Autodesk Inventor part; units mm, degrees
ref_plane "ba2_XY" through (19.05, 7.8105, 0) normal (0, 0, 1) x (1, 0, 0)
ref_plane "ba2_YZ" through (19.05, 7.8105, 0) normal (1, 0, 0) x (0, 1, 0)
ref_plane "ba2_ZX" through (19.05, 7.8105, 0) normal (0, 1, 0) x (0, 0, 1)
sketch "Sketch_1" plane through (0, 0, 0) normal (0, 0, 1) x (1, 0, 0)
  line L0 (29.3624, 0) -> (0, 0)
  line L1 (0, 0) -> (0, 6.7691)
  line L2 (0, 6.7691) -> (0.508, 7.2771)
  line L3 (0.508, 7.2771) -> (2.7432, 7.2771)
  line L4 (2.7432, 7.2771) -> (3.3782, 6.6421)
  line L5 (3.3782, 6.6421) -> (4.0132, 6.6421)
  line L6 (4.0132, 6.6421) -> (4.0132, 7.8105)
  line L7 (4.0132, 7.8105) -> (25.3492, 7.8105)
  line L8 (25.3492, 7.8105) -> (25.3492, 6.6421)
  line L9 (25.3492, 6.6421) -> (25.9842, 6.6421)
  line L10 (25.9842, 6.6421) -> (26.6192, 7.2771)
  line L11 (26.6192, 7.2771) -> (28.8544, 7.2771)
  line L12 (28.8544, 7.2771) -> (29.3624, 6.7691)
  line L13 (29.3624, 6.7691) -> (29.3624, 0)
  line L14 (29.3624, 0) -> (0, 0)
revolve "Revolution1" add sketch "Sketch_1" angle 360 about axis through (29.3624, 0, 0) along (1, 0, 0)
sketch "Sketch2" plane through (29.3624, 0, 0) normal (1, 0, 0) x (0, 0, -1)
  point P0 (0, 0)
hole "Hole1" at (29.3624, 0, 0) direction (-1, 0, 0) diameter 5.334 depth 29.3624
sketch "Sketch_6" plane through (0, 0, 0) normal (0, 0, 1) x (1, 0, 0)
  line L0 (19.05, 0) -> (19.05, 7.8105)
  line L1 (19.05, 7.8105) -> (23.0124, 7.8105)
  line L2 (23.0124, 7.8105) -> (23.0124, 6.7945)
  line L3 (23.0124, 6.7945) -> (21.463, 6.7945)
  line L4 (21.463, 6.7945) -> (21.0337, 6.3652)
  line L5 (21.0337, 6.3652) -> (21.0337, 0)
  line L6 (21.0337, 0) -> (19.05, 0)
  line L7 (19.05, 0) -> (19.05, 7.8105)
revolve "Revolution2" cut sketch "Sketch_6" angle 360 about axis through (19.05, 0, 0) along (0, -1, 0)
thread "Thread1"
sketch "Sketch_8" plane through (0, 0, 0) normal (0, 0, 1) x (1, 0, 0)
  line L0 (29.3624, 0) -> (-29.3624, 0)
  line L1 (24.7988, 6.6421) -> (25.0862, 6.6421)
  line L2 (25.0862, 6.6421) -> (26.1874, 7.7433)
  line L3 (26.1874, 7.7433) -> (26.1874, 7.8105)
  line L4 (26.1874, 7.8105) -> (25.9672, 7.8105)
  line L5 (25.9672, 7.8105) -> (24.7988, 6.6421)
revolve "Revolution3" add sketch "Sketch_8" angle 360 about axis through (29.3624, 0, 0) along (1, 0, 0)
sketch "Sketch_14" plane through (0, 0, 0) normal (0, 0, 1) x (1, 0, 0)
  line L0 (29.3624, 0) -> (-29.3624, 0)
  line L1 (3.175, 7.7433) -> (4.2762, 6.6421)
  line L2 (4.2762, 6.6421) -> (4.5636, 6.6421)
  line L3 (4.5636, 6.6421) -> (3.3952, 7.8105)
  line L4 (3.3952, 7.8105) -> (3.175, 7.8105)
  line L5 (3.175, 7.8105) -> (3.175, 7.7433)
revolve "Revolution4" add sketch "Sketch_14" angle 360 about axis through (29.3624, 0, 0) along (1, 0, 0)
ref_plane "ba2_XY" through (19.05, 7.8105, 0) normal (0, 0, 1) x (1, 0, 0)
ref_plane "ba2_YZ" through (19.05, 7.8105, 0) normal (1, 0, 0) x (0, 1, 0)
ref_plane "ba2_ZX" through (19.05, 7.8105, 0) normal (0, 1, 0) x (0, 0, 1)
ref_plane "centar_XY" through (14.6812, 0, 0) normal (1, 0, 0) x (0, 0, -1)
ref_plane "centar_YZ" through (14.6812, 0, 0) normal (0, 0, -1) x (0, 1, 0)
ref_plane "centar_ZX" through (14.6812, 0, 0) normal (0, 1, 0) x (1, 0, 0)
ref_plane "d1_XY" through (21.463, 6.7945, 0) normal (0, 0, 1) x (1, 0, 0)
ref_plane "d1_YZ" through (21.463, 6.7945, 0) normal (1, 0, 0) x (0, 1, 0)
ref_plane "d1_ZX" through (21.463, 6.7945, 0) normal (0, 1, 0) x (0, 0, 1)
ref_plane "d2_XY" through (16.637, 6.7945, 0) normal (0, 0, 1) x (1, 0, 0)
ref_plane "d2_YZ" through (16.637, 6.7945, 0) normal (1, 0, 0) x (0, 1, 0)
ref_plane "d2_ZX" through (16.637, 6.7945, 0) normal (0, 1, 0) x (0, 0, 1)
ref_plane "to_cyl_A_XY" through (2.7432, 0, 0) normal (1, 0, 0) x (0, 0, -1)
ref_plane "to_cyl_A_YZ" through (2.7432, 0, 0) normal (0, 0, -1) x (0, 1, 0)
ref_plane "to_cyl_A_ZX" through (2.7432, 0, 0) normal (0, 1, 0) x (1, 0, 0)
ref_plane "to_cyl_B_XY" through (26.6192, 0, 0) normal (1, 0, 0) x (0, 0, -1)
ref_plane "to_cyl_B_YZ" through (26.6192, 0, 0) normal (0, 0, -1) x (0, 1, 0)
ref_plane "to_cyl_B_ZX" through (26.6192, 0, 0) normal (0, 1, 0) x (1, 0, 0)
ref_plane "to_rod_A_XY" through (29.3624, 0, 0) normal (1, 0, 0) x (0, 0, -1)
ref_plane "to_rod_A_YZ" through (29.3624, 0, 0) normal (0, 0, -1) x (0, 1, 0)
ref_plane "to_rod_A_ZX" through (29.3624, 0, 0) normal (0, 1, 0) x (1, 0, 0)
properties part number "D-68355---0"
The model under review builds one solid part; all positions refer to its coordinate system, in mm. A direction names the side the tool comes from. Coordinates: 2 decimals unless noted, no trailing zeros. Loops run counter-clockwise (first coordinate to the right, second up) from the corner with the lowest first, then second, coordinate; pieces in that order, holes last. Notation, with made-up numbers: (15.5, 80.25) -> (36.5, 80.25) arc R12 cw to (36.5, 84.25) -> close; hole circle Ø3 at (0, 27.5). An arc over 180 degrees is marked (long way). Use a Markdown table: item, result. Add a question column.
1. To check wall thickness, follow line 1 (Z direction, x = 7, y = 0); line 2 (X direction, y = 3.55, z = 0); line 3 (Z direction, x = 19.05, y = 3.9). State the ranges of each line that lie inside material, in increasing order.
2. Clearance check with flat-ended pins moving along their axes: pin 1 Ø1 at (x, z) = (19, -2.5) entering from -Y; pin 2 Ø4 at (x, y) = (8, 3) entering from +Z. State where each tip first meets the part, or that it passes through.
3. Add section B-B on x = 8.25. Write out the cut boundary in (y, z).
4. Add section C-C on z = 0. Give the number of separate pieces and of enclosed holes in the cut face, plus the area to 3 significant figures.
5. Draft analysis for pull direction Y (two halves, no side actions). For faces 6 (the face through (0, 0, -3)), 7 (the face through (14.476, -2.644, 0.347)), 8 (the face through (21, 6.794, 2)), state which applies: pulls with the +Y half, pulls with the -Y half, needs draft (parallel to the pull), parting line crosses it, or undercut.
6. Add section A-A on x = 19.05. Write out the cut boundary in (y, z).
7. Machinability: for faces 1 (the face through (23.01, 7.18, -0.07)), 2 (the face through (14.831, -7.803, 0.343)), 3 (the face through (1.64, 6.94, 2.19)), 4 (the face through (27.75, 6.94, 2.19)), 5 (the face through (25.671, -1.44, -6.484)), which of the approach directions +Z, -Z, +X, -X, +Y, -Y give a long, thin tool a straight path to every point of the face, cutting with its end or side? Answer none if there is none.
Returned:
| question | item | result |
|---|---|---|
| 1 | line 1 | z = -7.81 to -2.67, 2.67 to 7.81 |
| 1 | line 2 | x = 0 to 17.07, 21.03 to 29.36 |
| 1 | line 3 | z = -6.77 to -1.98, 1.98 to 6.77 |
| 2 | pin 1 | stops at y = -7.55 |
| 2 | pin 2 | stops at z = 7.75 |
| 3 | outline | circle Ø15.62 at (0, 0); hole circle Ø5.33 at (0, 0) |
| 4 | separate pieces | 3 |
| 4 | enclosed holes | 0 |
| 4 | area | 267 mm² |
| 5 | face 6 | needs draft |
| 5 | face 7 | undercut |
| 5 | face 8 | pulls with the +Y half |
| 6 | outline | (1.78, -1.98) arc R2.67 cw (long way) to (1.78, 1.98) -> (6.37, 1.98) -> (6.79, 2.41) -> (6.79, 3.85) arc R7.81 ccw (long way) to (6.79, -3.85) -> (6.79, -2.41) -> (6.37, -1.98) -> close |
| 7 | face 1 | +Y |
| 7 | face 2 | +X, -X |
| 7 | face 3 | -X |
| 7 | face 4 | +X |
| 7 | face 5 | none |
